Model file for the job. Use its own axes, mm. Coordinates: 2 decimals unless noted, no trailing zeros. Loops run counter-clockwise (first coordinate to the right, second up) from the corner with the lowest first, then second, coordinate; pieces in that order, holes last.
from build123d import *

# Parameters (mm, degrees)
F1_DEPTH = 6
F2_R     = 4
F4_DEPTH = 6
F6_DEPTH = 6.001
F7_R     = 3
F8_R     = 0.5


with BuildPart() as f1:
    # F0 (on Front) → F1 (new body)
    with BuildSketch(Plane.XZ):
        with BuildLine():
            ThreePointArc((12, 31.5), (6.98702, 15.373992), (0, 0))
            Line((0, 0), (195, 0))
            ThreePointArc((195, 0), (199.533116, 25.594396), (202, 51.469805))
            Line((202, 51.469805), (12, 31.5))
        make_face()
    extrude(amount=F1_DEPTH)

    # F2
    f2_edges = [f1.edges().sort_by_distance(p)[0] for p in [
        (0, -3, 0),
        (195, -3, 0),
        (202, -3, 51.469805),
    ]]
    fillet(f2_edges, radius=F2_R)

    # F3 (on Front) → F4 (join)
    with BuildSketch(Plane.XZ):
        with BuildLine():
            ThreePointArc((14.934146, 47.896524), (13.7202, 39.652965), (12, 31.5))
            Line((12, 31.5), (27.724132, 33.152673))
            Line((27.724132, 33.152673), (28.857453, 49.359922))
            Line((28.857453, 49.359922), (14.934146, 47.896524))
        make_face()
    extrude(amount=F4_DEPTH)

    # F5 (on face) → F6 (cut, through all)
    with BuildSketch(Plane.XZ.offset(6)):
        with BuildLine():
            Line((141, 14.450166), (141, 29.549834))
            ThreePointArc((141, 29.549834), (133, 33), (125, 29.549834))
            Line((125, 29.549834), (125, 14.450166))
            ThreePointArc((125, 14.450166), (133, 11), (141, 14.450166))
        make_face()
    extrude(amount=-F6_DEPTH, mode=Mode.SUBTRACT)

    # F7
    f7_edges = [f1.edges().sort_by_distance(p)[0] for p in [
        (14.934146, -3, 47.896524),
        (28.857453, -3, 49.359922),
        (27.724132, -3, 33.152673),
        (125, -3, 14.450166),
        (125, -3, 29.549834),
        (141, -3, 29.549834),
        (141, -3, 14.450166),
    ]]
    fillet(f7_edges, radius=F7_R)

    # F8
    f8_edges = [f1.edges().sort_by_distance(p)[0] for p in [
        (10.297784, -6, 25.178986),
        (10.297784, 0, 25.178986),
    ]]
    fillet(f8_edges, radius=F8_R)


solid = f1.part
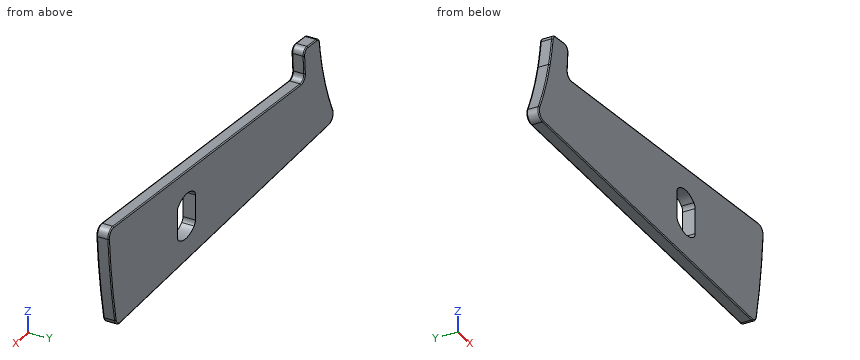
Q1. Flat gauge pin, fed straight in: P1, Ø1.8, axis at y = -3.5, z = 22.5, coming from the -X side. Where does the tip first touch, or does it go through?
Answers:
P1: stops at x = 9.19
Q2. Drill centre lines: line 1 (X direction, y = -3.5, z = 16); line 2 (X direction, y = -5, z = 17); line 3 (Z direction, x = 182.5, y = -4.25). Where is each one in solid material? Low to high.
Answers:
line 1: x = 7.22 to 125, 141 to 198.08
line 2: x = 7.59 to 125, 141 to 198.25
line 3: z = 0 to 49.42
Q3. Slice it at A-A (y = -3.5). List the corners of the cut face in (x, z) (3 decimals).
Answers:
outline: (2.868, 5.71) arc R4 ccw to (6.484, 0) - (191.764, 0) arc R4 ccw to (195.68, 3.184) arc R324 ccw to (201.704, 46.719) arc R4 ccw to (197.295, 50.975) - (31.28, 33.526) arc R3 cw to (27.974, 36.719) - (28.608, 45.793) arc R3 ccw to (25.302, 48.986) - (17.303, 48.145) arc R3 ccw to (14.643, 45.559) arc R135 cw to (12, 31.5) arc R135 cw to start; hole (125, 15.755) arc R3 ccw to (126.125, 13.413) arc R11 ccw to (139.875, 13.413) arc R3 ccw to (141, 15.755) - (141, 28.245) arc R3 ccw to (139.875, 30.587) arc R11 ccw to (126.125, 30.587) arc R3 ccw to (125, 28.245) - close
